Build history of the part. All positions in model axes, mm. A direction names the side the tool comes from. Round coordinates to 2 decimals unless told otherwise and drop trailing zeros. Write each loop counter-clockwise with the first axis right and the second up, starting at its lowest first coordinate (ties: lowest second). Pieces come first, ordered by that corner, then holes.
1) Saw through at B-B (y = 2.75). Write the cut outline in (x, z), plus the area to 3 significant figures.
2) Saw through at C-C (z = 7.5). Write the cut outline in (x, y).
3) Saw through at D-D (x = 0). Write the cut outline in (y, z), plus the area to 3 significant figures.
4) Which spindle directions (+Z, -Z, +X, -X, +Y, -Y) get a long thin tool onto all of the face, cutting with end or side? Do faces 1 (the flat face through (1, -2, 3.5)), 2 (the flat face through (0, 0, 14)). Say none if no direction does.
5) Saw through at A-A (x = -4.5). Write the cut outline in (y, z).
6) Wall check: probe 1 along Z at (x, y) = (-2, 4.75); probe 2 along Z at (x, y) = (-1.25, 2.25); probe 3 along Y at (x, z) = (1.5, 5.5). Give the ranges that are in metal, low to high.
7) Flat gauge pins, fed straight in: pin 1 (5 mm diameter, centred on y = 2, z = 10, fed in from +X); pin 2 (5 mm diameter, centred on x = -3.5, z = 8, fed in from +Y). Where does each tip first touch, or does it go through?
from build123d import *

# Parameters (mm, degrees)
SKETCH1_W           = 11
SKETCH1_H           = 11
BOSS_EXTRUDE1_DEPTH = 2
SKETCH2_R           = 2
BOSS_EXTRUDE2_DEPTH = 12
CHAMFER1_SIZE       = 0.1
SKETCH3_R           = 3
BOSS_EXTRUDE3_DEPTH = 1.5
CHAMFER2_SIZE       = 0.5


with BuildPart() as part:
    # Sketch1 → Boss-Extrude1 (new body)
    with BuildSketch(Plane.XY):
        Rectangle(SKETCH1_W, SKETCH1_H)
    extrude(amount=BOSS_EXTRUDE1_DEPTH)

    # Sketch2 → Boss-Extrude2 (add)
    with BuildSketch(Plane.XY.offset(2)):
        Circle(SKETCH2_R)
    extrude(amount=BOSS_EXTRUDE2_DEPTH)

    # Chamfer1
    chamfer1_edges = [part.edges().sort_by_distance(p)[0] for p in [
        (-5.5, 0, 2),
        (0, -5.5, 2),
        (5.5, 0, 2),
        (0, -5.5, 0),
        (-5.5, 0, 0),
        (0, 5.5, 0),
        (5.5, 0, 0),
        (0, 5.5, 2),
        (-5.5, 5.5, 1),
        (5.5, 5.5, 1),
    ]]
    chamfer(chamfer1_edges, length=CHAMFER1_SIZE)

    # Sketch3 → Boss-Extrude3 (add)
    with BuildSketch(Plane.XY.offset(2)):
        Circle(SKETCH3_R)
    extrude(amount=BOSS_EXTRUDE3_DEPTH)

    # Chamfer2
    chamfer2_edges = [part.edges().sort_by_distance(p)[0] for p in [
        (-2, 0, 14),
    ]]
    chamfer(chamfer2_edges, length=CHAMFER2_SIZE)


solid = part.part
Evaluation:
1. outline: (-5.5, 0.1) - (-5.4, 0) - (5.4, 0) - (5.5, 0.1) - (5.5, 1.9) - (5.4, 2) - (1.2, 2) - (1.2, 3.5) - (-1.2, 3.5) - (-1.2, 2) - (-5.4, 2) - (-5.5, 1.9) - close
1. area: 25.6 mm2
2. outline: circle Ø4 at (0, 0)
3. outline: (-5.5, 0.1) - (-5.4, 0) - (5.4, 0) - (5.5, 0.1) - (5.5, 1.9) - (5.4, 2) - (3, 2) - (3, 3.5) - (2, 3.5) - (2, 13.5) - (1.5, 14) - (-1.5, 14) - (-2, 13.5) - (-2, 3.5) - (-3, 3.5) - (-3, 2) - (-5.4, 2) - (-5.5, 1.9) - close
3. area: 72.7 mm2
4. face 1: +Z
4. face 2: +Z, +X, -X, +Y, -Y
5. outline: (-5.5, 0.1) - (-5.4, 0) - (5.4, 0) - (5.5, 0.1) - (5.5, 1.9) - (5.4, 2) - (-5.4, 2) - (-5.5, 1.9) - close
6. probe 1: z = 0 to 2
6. probe 2: z = 0 to 3.5
6. probe 3: y = -1.32 to 1.32
7. pin 1: stops at x = 2
7. pin 2: stops at y = 1.73
